```python
from build123d import *

# Parameters (mm, degrees)
ESBO_O2_W                = 100
ESBO_O2_H                = 100
ESBO_O2_W_2              = 96
ESBO_O2_H_2              = 96
RESSALTO_EXTRUS_O1_DEPTH = 2
ESBO_O2_3_W              = 96
ESBO_O2_3_H              = 96
RESSALTO_EXTRUS_O2_DEPTH = 5.7
FILETE2_R                = 2
ESBO_O4_R                = 7.5
ESBO_O4_R_2              = 1.65
CORTE_EXTRUS_O1_DEPTH    = 142.53617912


with BuildPart() as part:
    # Esbo_o2 → Ressalto-extrus_o1 (new body)
    # profile 1 of 2: a face of its own
    with BuildSketch(Plane(origin=(0, 0, 0), x_dir=(1, 0, 0), z_dir=(0, 1, 0))):
        with Locations((50, 50)):
            Rectangle(ESBO_O2_W, ESBO_O2_H)
        with Locations((50, 50)):
            Rectangle(ESBO_O2_W_2, ESBO_O2_H_2, mode=Mode.SUBTRACT)
    # profile 2 of 2: a face of its own
    with BuildSketch(Plane(origin=(0, 0, 0), x_dir=(1, 0, 0), z_dir=(0, 1, 0))):
        with Locations((50, 50)):
            Rectangle(ESBO_O2_W_2, ESBO_O2_H_2)
    extrude(amount=RESSALTO_EXTRUS_O1_DEPTH)

    # Esbo_o2_3 → Ressalto-extrus_o2 (add)
    with BuildSketch(Plane(origin=(0, 0, 0), x_dir=(1, 0, 0), z_dir=(0, 1, 0))):
        with Locations((50, 50)):
            Rectangle(ESBO_O2_3_W, ESBO_O2_3_H)
    extrude(amount=RESSALTO_EXTRUS_O2_DEPTH)

    # Filete2
    filete2_edges = [part.edges().sort_by_distance(p)[0] for p in [
        (2, 3.85, -2),
        (98, 3.85, -2),
        (98, 3.85, -98),
        (2, 3.85, -98),
        (0, 1, 0),
        (0, 1, -100),
        (100, 1, -100),
        (100, 1, 0),
    ]]
    fillet(filete2_edges, radius=FILETE2_R)

    # Esbo_o4 → Corte-extrus_o1 (cut, through all)
    with BuildSketch(Plane(origin=(0, 0, 0), x_dir=(1, 0, 0), z_dir=(0, 1, 0))):
        with Locations(Location((50, 50, 0), (0, 0, 270))):
            Circle(ESBO_O4_R)
        with Locations(Location((50, 25, 0), (0, 0, 270))):
            Circle(ESBO_O4_R_2)
        with Locations(Location((28.349364905, 62.5, 0), (0, 0, 270))):
            Circle(ESBO_O4_R_2)
        with Locations(Location((71.650635095, 62.5, 0), (0, 0, 270))):
            Circle(ESBO_O4_R_2)
    extrude(amount=CORTE_EXTRUS_O1_DEPTH, mode=Mode.SUBTRACT)


solid = part.part
```
The model under review builds one solid part; all positions refer to its coordinate system, in mm. A direction names the side the tool comes from. Round coordinates to 2 decimals unless told otherwise and drop trailing zeros. Order: outer loops, then holes, each group sorted by start corner. A loop starts at its lowest first (then second) coordinate and runs counter-clockwise, first axis right, second up.
(1) For P1, Ø1.8, axis at x = 39.5, y = 4, coming from the +Z side; P2, Ø3, axis at x = 70.5, y = 2.5, coming from the +Z side; P3, Ø1.8, axis at y = 3, z = -42.5, coming from the +X side; P4, Ø1.1, axis at y = 3, z = -60, coming from the -X side, all flat-tipped, find the tip position at first contact; note any pin that passes through.
Working result:
P1: stops at z = -2
P2: stops at z = 0
P3: stops at x = 98
P4: stops at x = 2
(2) Mouldability with a two-part tool opening along X and no side actions: class faces 6 (the face through (98, 4, -49)), 7 (the face through (72.766, 2.81, -63.716)), 8 (the face through (1.6, 2, -72.5)) as released by +X, released by -X, zero draft, split by the parting line, or undercut.
Working result:
face 6: released by +X
face 7: undercut
face 8: zero draft
(3) Take a section at C-C, the plane z = -50. State the section outline as (x, y) points, plus the area to 3 significant figures.
Working result:
outline: (0, 0) - (42.5, 0) - (42.5, 5.7) - (2, 5.7) - (2, 2) - (0, 2) - close; (57.5, 0) - (100, 0) - (100, 2) - (98, 2) - (98, 5.7) - (57.5, 5.7) - close
area: 470 mm2
(4) Take a section at B-B, the plane x = 50. State the section outline as (y, z) points.
Working result:
outline: (0, -100) - (2, -100) - (2, -98) - (5.7, -98) - (5.7, -57.5) - (0, -57.5) - close; (0, -42.5) - (5.7, -42.5) - (5.7, -26.65) - (0, -26.65) - close; (0, -23.35) - (5.7, -23.35) - (5.7, -2) - (2, -2) - (2, 0) - (0, 0) - close
(5) Take a section at A-A, the plane z = -62.5. State the section outline as (x, y) points.
Working result:
outline: (0, 0) - (26.7, 0) - (26.7, 5.7) - (2, 5.7) - (2, 2) - (0, 2) - close; (30, 0) - (70, 0) - (70, 5.7) - (30, 5.7) - close; (73.3, 0) - (100, 0) - (100, 2) - (98, 2) - (98, 5.7) - (73.3, 5.7) - close
(6) Take a section at D-D, the plane y = 1. State the section outline as (x, z) points, plus the area to 3 significant figures.
Working result:
outline: (0, -98) arc R2 ccw to (2, -100) - (98, -100) arc R2 ccw to (100, -98) - (100, -2) arc R2 ccw to (98, 0) - (2, 0) arc R2 ccw to (0, -2) - close; hole circle Ø3.3 at (28.35, -62.5); hole circle Ø15 at (50, -50); hole circle Ø3.3 at (50, -25); hole circle Ø3.3 at (71.65, -62.5)
area: 9,790 mm2
(7) Tool access review of faces 1 (the face through (49, 4, -2)), 2 (the face through (2, 4, -49)), 3 (the face through (49, 0, -40)), 4 (the face through (51.115, 2.81, -26.216)), 5 (the face through (49, 4, -98)): name each direction out of +Z, -Z, +X, -X, +Y, -Y from which nothing blocks a thin tool from reaching the whole face with its end or side.
Working result:
face 1: +Z, +X, -X, +Y
face 2: +Z, -Z, -X, +Y
face 3: +Z, -Z, +X, -X, -Y
face 4: +Y, -Y
face 5: -Z, +X, -X, +Y
(8) Wall thickness on L1, parallel to X at y = 3.4, z = -62.5; L2, parallel to X at y = 1.85, z = -62.5; L3, parallel to Z at x = 50, y = 4.45: over which ranges is each line inside the solid? List them lowest first.
Working result:
L1: x = 2 to 26.7, 30 to 70, 73.3 to 98
L2: x = 0 to 26.7, 30 to 70, 73.3 to 100
L3: z = -98 to -57.5, -42.5 to -26.65, -23.35 to -2
